Geometry: final body of the model. Coordinates: model frame, mm. A direction names the side the tool comes from. Give positions to 0.01 mm unless a question says otherwise; leave off trailing zeros. Order: outer loops, then holes, each group sorted by start corner. A loop starts at its lowest first (then second) coordinate and runs counter-clockwise, first axis right, second up. Notation, with made-up numbers: (31.25, 59.25) -> (43.25, 59.25) arc R18 ccw to (43.25, 76.25) -> close; hole circle Ø11 at (11, 56.25). An arc over 180 degrees is marked (long way). Answer in a Markdown table with one row per item. Add a question column.
Q1. Line query: line 1 along X through (y, z) = (0.7, 25.4) (3 decimals); line 2 along X through (y, z) = (0.25, 23) (3 decimals); line 3 along Z through (x, y) = (-18, 2.8). Output: solid intervals per line, ascending. Write a range as from..to.
Q2. Set-up query: faces 4 (the face through (12.065, 2, 25)), 5 (the face through (-24, 2, 30.162)), 6 (the face through (-22.4, 1.6, -4.1)). Return all of +Z, -Z, +X, -X, +Y, -Y with unobstructed straight access to the full face (end or side cutting, diameter ignored); none if empty.
Q3. Pull-direction query (X, two-part tool) for faces 1 (the face through (22, 2, 30.162)), 2 (the face through (-17.68, 1.57, 26.9)), 3 (the face through (31.297, 1.61, 29.685)); classes: +X half, -X half, draft (parallel to the pull), parting line (faces both ways), or undercut.
Q4. Cut plane A-A on z = 25.4. Return the cut outline in (x, y) (3 decimals).
Q5. Cut plane D-D on x = 19.05. Return the cut outline in (y, z) (1 decimal).
Q6. Cut plane B-B on y = 1.55. Count the separate pieces of the cut face and the enclosed holes in it, and give its area (3 significant figures).
Q7. Cut plane C-C on z = -5.5. Return the cut outline in (x, y) (3 decimals), and give its area (3 significant figures).
from build123d import *

# Parameters (mm, degrees)
SKETCH1_W           = 63.5
SKETCH1_H           = 60.325
BOSS_EXTRUDE1_DEPTH = 3.175
SKETCH2_R           = 2.032
CUT_EXTRUDE1_DEPTH  = 44.908080478
SKETCH3_W           = 28.575
SKETCH3_H           = 9.652
CUT_EXTRUDE2_DEPTH  = 44.908080478
FILLET1_R           = 1.5875
CUT_EXTRUDE4_DEPTH  = 44.908080478
FILLET2_R           = 1.27


with BuildPart() as part:
    # Sketch1 → Boss-Extrude1 (new body)
    with BuildSketch(Plane(origin=(0, 0, 0), x_dir=(1, 0, 0), z_dir=(0, 1, 0))):
        Rectangle(SKETCH1_W, SKETCH1_H)
    extrude(amount=BOSS_EXTRUDE1_DEPTH)

    # Sketch2 → Cut-Extrude1 (cut, through all)
    with BuildSketch(Plane(origin=(0, 0, 0), x_dir=(-1, 0, 0), z_dir=(0, -1, 0))):
        with Locations(Location((-19.05, -25.4, 0), (0, 0, 90))):
            Circle(SKETCH2_R)
        with Locations(Location((19.05, -25.4, 0), (0, 0, 90))):
            Circle(SKETCH2_R)
    extrude(amount=-CUT_EXTRUDE1_DEPTH, mode=Mode.SUBTRACT)

    # Sketch3 → Cut-Extrude2 (cut, through all)
    with BuildSketch(Plane(origin=(0, 3.175, 0), x_dir=(1, 0, 0), z_dir=(0, 1, 0))):
        with Locations((-2.2225, -25.3365)):
            Rectangle(SKETCH3_W, SKETCH3_H)
    extrude(amount=-CUT_EXTRUDE2_DEPTH, mode=Mode.SUBTRACT)

    # Fillet1
    fillet1_edges = [part.edges().sort_by_distance(p)[0] for p in [
        (-16.51, 1.5875, 30.1625),
        (-16.51, 1.5875, 20.5105),
        (12.065, 1.5875, 20.5105),
        (12.065, 1.5875, 30.1625),
        (31.75, 1.5875, 30.1625),
        (-31.75, 1.5875, 30.1625),
    ]]
    fillet(fillet1_edges, radius=FILLET1_R)

    # Sketch5 → Cut-Extrude4 (cut, through all)
    with BuildSketch(Plane(origin=(0, 3.175, 0), x_dir=(1, 0, 0), z_dir=(0, 1, 0))):
        with BuildLine():
            Line((-15.24, -1.27), (-31.75, 11.1125))
            Line((-31.75, 11.1125), (-31.75, 30.1625))
            Line((-31.75, 30.1625), (31.75, 30.1625))
            Line((31.75, 30.1625), (23.603733945, 9.667903014))
            ThreePointArc((23.603733945, 9.667903014), (6.884580014, -5.399183177), (-15.24, -1.27))
        make_face()
    extrude(amount=-CUT_EXTRUDE4_DEPTH, mode=Mode.SUBTRACT)

    # Fillet2
    fillet2_edges = [part.edges().sort_by_distance(p)[0] for p in [
        (31.75, 1.5875, -30.1625),
        (-31.75, 1.5875, -11.1125),
    ]]
    fillet(fillet2_edges, radius=FILLET2_R)


solid = part.part
Completed:
| question | item | result |
|---|---|---|
| 1 | line 1 | x = -31.75..-21.082, -17.018..-16.51, 12.065..17.018, 21.082..31.75 |
| 1 | line 2 | x = -31.75..-16.51, 12.065..31.75 |
| 1 | line 3 | z = -0.8..23.66, 27.14..30.16 |
| 2 | face 4 | +Z, +Y, -Y |
| 2 | face 5 | +Z, +X, -X, +Y, -Y |
| 2 | face 6 | -Z, +Y, -Y |
| 3 | face 1 | draft |
| 3 | face 2 | undercut |
| 3 | face 3 | +X half |
| 4 | outline | (-31.75, 0) -> (-21.082, 0) -> (-21.082, 3.175) -> (-31.75, 3.175) -> close; (-17.018, 0) -> (-16.51, 0) -> (-16.51, 3.175) -> (-17.018, 3.175) -> close; (12.065, 0) -> (17.018, 0) -> (17.018, 3.175) -> (12.065, 3.175) -> close; (21.082, 0) -> (31.75, 0) -> (31.75, 3.175) -> (21.082, 3.175) -> close |
| 5 | outline | (0, -2.2) -> (3.2, -2.2) -> (3.2, 23.4) -> (0, 23.4) -> close; (0, 27.4) -> (3.2, 27.4) -> (3.2, 30.2) -> (0, 30.2) -> close |
| 6 | separate pieces | 1 |
| 6 | enclosed holes | 2 |
| 6 | area | 1,730 mm² |
| 7 | outline | (-31.75, 0) -> (-24.267, 0) -> (-24.267, 3.175) -> (-31.75, 3.175) -> close; (21.484, 0) -> (31.75, 0) -> (31.75, 3.175) -> (21.484, 3.175) -> close |
| 7 | area | 56.4 mm² |
